from build123d import *

# Parameters (mm, degrees)
FILLET_1_R               = 0.5
SKETCH_11_R              = 2.05
CUT_EXTRUDE_3_DEPTH      = 3
CUT_EXTRUDE_6_DEPTH      = 6
CUT_EXTRUDE_6_DEPTH_BACK = 36.24556726
SKETCH_13_R              = 1.75
CUT_EXTRUDE_7_DEPTH      = 1
SKETCH_16_R              = 2
CUT_EXTRUDE_8_DEPTH      = 1


with BuildPart() as part:
    # 草图2 → 旋转1 (revolve)
    with BuildSketch(Plane.XY, mode=Mode.PRIVATE) as revolve_1_sk:
        with BuildLine():
            Line((7, 2), (7, 0))
            Line((7, 0), (24, 0))
            Line((24, 0), (24, 11.5))
            Line((24, 11.5), (22, 11.5))
            Line((22, 11.5), (22, 10.846618531))
            ThreePointArc((22, 10.846618531), (22.804161855, 10.074709263), (23.1, 9))
            ThreePointArc((23.1, 9), (22.804161855, 7.925290737), (22, 7.153381469))
            Line((22, 7.153381469), (22, 2))
            Line((22, 2), (7, 2))
        make_face()
    revolve(revolve_1_sk.sketch.rotate(Axis((0, 2, 0), (0, -1, 0)), 180), axis=Axis((0, 2, 0), (0, -1, 0)))

    # 圆角1
    fillet_1_edges = [part.edges().sort_by_distance(p)[0] for p in [
        (24, 11.5, 0),
        (24, 0, 0),
    ]]
    fillet(fillet_1_edges, radius=FILLET_1_R)

    # 草图11 → 切除-拉伸3 (cut)
    with BuildSketch(Plane(origin=(0, 11.5, 0), x_dir=(1, 0, 0), z_dir=(0, 1, 0))):
        with Locations((-21, 0)):
            Circle(SKETCH_11_R)
    extrude(amount=-CUT_EXTRUDE_3_DEPTH, mode=Mode.SUBTRACT)

    # 草图13 → 切除-拉伸6 (cut, two sides: drawn at the far end of the back side and taken through both)
    with BuildSketch(Plane(origin=(0, 2, 0), x_dir=(1, 0, 0), z_dir=(0, 1, 0)).offset(-CUT_EXTRUDE_6_DEPTH_BACK)):
        with Locations(Location((-21, 0, 0), (0, 0, 122.913164288))):
            Circle(SKETCH_13_R)
    extrude(amount=CUT_EXTRUDE_6_DEPTH + CUT_EXTRUDE_6_DEPTH_BACK, mode=Mode.SUBTRACT)

    # 草图15 → 切除-拉伸7 (cut)
    with BuildSketch(Plane(origin=(0, 2, 0), x_dir=(1, 0, 0), z_dir=(0, 1, 0))):
        Polygon((-2.833161507, 15.5), (-1.216580754, 18.3), (2.016580754, 18.3), (3.633161507, 15.5), (2.016580754, 12.7), (-1.216580754, 12.7), align=None)
        Polygon((2.016580754, -12.7), (-1.216580754, -12.7), (-2.833161507, -15.5), (-1.216580754, -18.3), (2.016580754, -18.3), (3.633161507, -15.5), align=None)
    extrude(amount=-CUT_EXTRUDE_7_DEPTH, mode=Mode.SUBTRACT)

    # 草图16 → 切除-拉伸8 (cut)
    with BuildSketch(Plane(origin=(0, 1, 0), x_dir=(1, 0, 0), z_dir=(0, 1, 0))):
        with Locations(Location((0.4, 15.5, 0), (0, 0, 270))):
            Circle(SKETCH_16_R)
        with Locations(Location((0.4, -15.5, 0), (0, 0, 270))):
            Circle(SKETCH_16_R)
    extrude(amount=-CUT_EXTRUDE_8_DEPTH, mode=Mode.SUBTRACT)


solid = part.part
Can you work these out from the model? Positions are in its coordinate system, mm. A direction names the side the tool comes from. Give positions to 0.01 mm unless a question says otherwise; leave off trailing zeros. Order: outer loops, then holes, each group sorted by start corner. A loop starts at its lowest first (then second) coordinate and runs counter-clockwise, first axis right, second up. Notation, with made-up numbers: M 38,1.5 L 86,1.5 A11 cw 86,22.5 Z; hole C -13.5,69 d3. An arc over 180 degrees is marked long. Use one line per item in the form item = value. Start each with the question number.
Item 1: If we section it at A-A (x = 0.4): State how many separate pieces and enclosed holes the cut face has, then the cut area to 3 significant figures.
Item 2: If we section it at B-B (y = 3.5): Write out the boundary of the cut face in (x, z).
Item 3: For faces 1 (the flat face through (2.836, 1.507, 14.12)), 2 (the cylindrical face through (-6.466, 0.986, 2.681)), which set-ups out of +Z, -Z, +X, -X, +Y, -Y let a thin tool reach every point of the face, with its end or its side?
Item 4: If I drill on line 1 along Z through (x, y) = (0, 11.05); line 2 along X through (y, z) = (7.5, 6.5); line 3 along Z through (x, y) = (2.5, 6.5), over which ranges is the centre line in solid material (lowest first)?
Item 5: Will these pins go through, and if not, where does the flat tip stop? pin 1 Ø3 at (y, z) = (5, -8.5) entering from -X; pin 2 Ø0.8 at (x, y) = (0.5, 1.5) entering from +Z; pin 3 Ø6 at (x, y) = (6, 9) entering from +Z; pin 4 Ø6.5 at (x, z) = (0.4, -15.5) entering from -Y.
Outcome:
q1.separate_pieces = 4
q1.enclosed_holes = 0
q1.area = 80.8 mm2
q2.outline = C 0,0 d48; hole M -21.95,-1.47 A22 ccw long -21.95,1.47 A1.75 ccw Z
q3.face_1 = +Y
q3.face_2 = +Y, -Y
q4.line_1 = -24 to -22, 22 to 24
q4.line_2 = -23.1 to -21.51, 21.51 to 23.1
q4.line_3 = -23.87 to -21.86, 21.86 to 23.87
q5.pin_1 = -22.96
q5.pin_2 = 24
q5.pin_3 = 23.81
q5.pin_4 = 0
